from build123d import *


with BuildPart() as part:
    # Sketch1 → Revolve1 (revolve)
    with BuildSketch(Plane.XY):
        with BuildLine():
            Line((39.587859575, 60.721319219), (39.587859575, 20.721319219))
            Line((39.587859575, 20.721319219), (34.15419798, 20.721319219))
            ThreePointArc((34.15419798, 20.721319219), (33.398410087, 20.376135729), (33.1643932, 19.578888541))
            Line((33.1643932, 19.578888541), (50, -97.418126201))
            ThreePointArc((50, -97.418126201), (52.679906162, -102.324983923), (57.918438238, -104.278680781))
            Line((57.918438238, -104.278680781), (70, -104.278680781))
            Line((70, -104.278680781), (70, -124.278680781))
            Line((70, -124.278680781), (50, -124.278680781))
            Line((50, -124.278680781), (50, -122.278680781))
            ThreePointArc((50, -122.278680781), (49.707106781, -121.571574), (49, -121.278680781))
            Line((49, -121.278680781), (43.330477707, -121.278680781))
            Line((43.330477707, -121.278680781), (35.697641886, -68.23521073))
            Line((35.697641886, -68.23521073), (25, 6.106758666))
            Line((25, 6.106758666), (25, 60.721319219))
            Line((25, 60.721319219), (39.587859575, 60.721319219))
        make_face()
    revolve(axis=Axis((0, 76.173744253, 0), (0, -1, 0)))


solid = part.part
Build history of the part. All positions in model axes, mm. A direction names the side the tool comes from. Coordinates: 2 decimals unless noted, no trailing zeros. Order: outer loops, then holes, each group sorted by start corner. A loop starts at its lowest first (then second) coordinate and runs counter-clockwise, first axis right, second up. Notation, with made-up numbers: M -16.5,85 L 0.5,85 A29 ccw 0.5,115 Z; hole C -28,88 d10. An arc over 180 degrees is marked long. One line per question, with ' | ' between items. Start each with the question number.
Q1. Two-plate mould, pull along X, no slides. Class faces 1 (the face through (-55.55, -114.419, -42.594)), 2 (the face through (-3.86, -121.279, -43.33)), 3 (the face through (-30, 20.721, -17)), 4 (the face through (47.69, -123.26, 15.02)): +X half, -X half, draft (parallel to the pull), parting line (faces both ways), or undercut.
Q2. Flat gauge pins, fed straight in: pin 1 Ø3 at (x, y) = (49.5, -79.5) entering from -Z; pin 2 Ø10 at (x, y) = (-16, 0.5) entering from +Z; pin 3 Ø8 at (x, y) = (-2, 12.5) entering from +Z; pin 4 Ø3 at (y, z) = (-14.5, -26) entering from +X. Where does each tip first touch, or does it go through?
Q3. Saw through at B-B (y = 10.5). List the corners of the cut face in (x, z), then the cut area to 3 significant figures.
Q4. 3-axis set-ups, long thin cutter, end or side, ignore diameter. For faces 5 (the face through (39.774, -39.739, 12.526)), 6 (the face through (26, -104.279, 52)), 7 (the face through (-26, 60.721, 1)): which of +Z, -Z, +X, -X, +Y, -Y reach the whole face in a straight line?
Q5. Saw through at A-A (y = 44.5). List the corners of the cut face in (x, z).
Q6. Probe L1, parallel to Z at x = 0, y = -123.45; L2, parallel to Z at x = 0, y = 21; L3, parallel to X at y = -13.5, z = 14. List the from-to ranges inside material, lowest first. Write a range as from..to.
Check values:
1) face 1: parting line | face 2: undercut | face 3: draft | face 4: undercut
2) pin 1: passes through | pin 2: stops at z = 34.35 | pin 3: stops at z = 34.73 | pin 4: stops at x = 29.17
3) outline: C 0,0 d68.94; hole C 0,0 d50 | area: 1,770 mm2
4) face 5: none | face 6: +Y | face 7: +Z, -Z, +X, -X, +Y
5) outline: C 0,0 d79.18; hole C 0,0 d50
6) L1: z = -70..-50, 50..70 | L2: z = -39.59..-25, 25..39.59 | L3: x = -35.25..-24.04, 24.04..35.25
